```python
from build123d import *

# Parameters (mm, degrees)
SKETCH1_W              = 200
SKETCH1_H              = 50
BOSS_EXTRUDE1_DEPTH    = 7.5
CUT_EXTRUDE1_DEPTH     = 105.16333328
SHELL2_T               = -2
F_20_0MM_DOWEL_HOLE1_D = 2.9


with BuildPart() as part:
    # Sketch1 → Boss-Extrude1 (new, symmetric)
    with BuildSketch(Plane.XY):
        Rectangle(SKETCH1_W, SKETCH1_H)
    extrude(amount=BOSS_EXTRUDE1_DEPTH, both=True)

    # Sketch15 → Cut-Extrude1 (cut, through all)
    with BuildSketch(Plane(origin=(0, 0, -7.5), x_dir=(-1, 0, 0), z_dir=(0, 0, -1))):
        Polygon((-100.000000026, 0.510192391), (-100, 25), (100, 25), (100.000000026, 0.510192391), (0, 20.08555215), align=None)
        Polygon((-100.000000029, -0.965448702), (-100, -25), (100, -25), (100, -0.965448702), (0, -20.08535521), align=None)
    extrude(amount=-CUT_EXTRUDE1_DEPTH, mode=Mode.SUBTRACT)

    # Shell2
    shell2_openings = [part.faces().sort_by_distance(p)[0] for p in [
        (4e-09, -0.078500046, -7.5),
    ]]
    offset(amount=SHELL2_T, openings=shell2_openings)

    # Ø20.0mm Dowel Hole1 (through all)
    with Locations(Plane.XY.offset(7.5)):
        with Locations((-11.490485194, 11.490485194), (11.490485194, -11.490485194), (11.490485194, 11.490485194), (-11.490485194, -11.490485194)):
            Hole(F_20_0MM_DOWEL_HOLE1_D / 2)


solid = part.part
```
Model file for the job. Use its own axes, mm. A direction names the side the tool comes from. Give positions to 0.01 mm unless a question says otherwise; leave off trailing zeros. Write each loop counter-clockwise with the first axis right and the second up, starting at its lowest first coordinate (ties: lowest second). Pieces come first, ordered by that corner, then holes. Notation, with made-up numbers: M 22.5,84.5 L 47.5,84.5 A20 cw 47.5,91.5 Z; hole C 8,36 d11. An arc over 180 degrees is marked long. Use a Markdown table: item, result.
1) Tool access for faces 4 (the flat face through (-1, 0, 7.5)), 5 (the flat face through (-47.295, -9.006, -1.091)): list every direction of +Z, -Z, +X, -X, +Y, -Y with a clear straight run to the whole face (end or side of a thin tool).
Responses:
| item | result |
|---|---|
| face 4 | +Z, +X, -X, +Y, -Y |
| face 5 | -Z |
2) Cut at B-B (y = 2.5). List the corners of the cut face in (x, z).
Responses:
| item | result |
|---|---|
| outline | M -89.84,-7.5 L -79.42,-7.5 L -79.42,5.5 L 79.42,5.5 L 79.42,-7.5 L 89.84,-7.5 L 89.84,7.5 L -89.84,7.5 Z |
3) Pin check, flat tips, straight feed: pin 1 (2 mm diameter, centred on x = 39.5, z = 0, fed in from +Y); pin 2 (1.7 mm diameter, centred on x = 11.49, y = 11.49, fed in from +Z); pin 3 (4.5 mm diameter, centred on x = -11.49, y = -11.49, fed in from -Z); pin 4 (3 mm diameter, centred on x = -10.5, z = 3.5, fed in from +Y). Stop position of each tip, or through.
Responses:
| item | result |
|---|---|
| pin 1 | stops at y = 12.55 |
| pin 2 | passes through |
| pin 3 | stops at z = 5.5 |
| pin 4 | stops at y = 18.32 |
4) Pull direction X, two halves, no side cores. Call faces 1 (the flat face through (-50.7, 10.16, -0.11)), 2 (the flat face through (-1, 0, 5.5)), 3 (the flat face through (7, -18, -7.5)): +X half, -X half, draft (parallel to the pull), parting line (faces both ways), or undercut.
Responses:
| item | result |
|---|---|
| face 1 | -X half |
| face 2 | undercut |
| face 3 | draft |
5) Cut at C-C (x = 29). List the corners of the cut face in (y, z).
Responses:
| item | result |
|---|---|
| outline | M -14.54,-7.5 L -12.5,-7.5 L -12.5,5.5 L 12.37,5.5 L 12.37,-7.5 L 14.41,-7.5 L 14.41,7.5 L -14.54,7.5 Z |
6) Cut at A-A (z = -0.5). List the corners of the cut face in (x, y).
Responses:
| item | result |
|---|---|
| outline | M -100,-0.97 L 0,-20.09 L 100,-0.97 L 100,0.51 L 0,20.09 L -100,0.51 Z; hole M -93.28,-0.21 L 0,-18.05 L 93.28,-0.21 L 0,18.05 Z |
7) Drill centre lines: line 1 (Z direction, x = 20, y = -6.5); line 2 (Y direction, x = 84, z = -4); line 3 (Y direction, x = -60, z = -6). Where is each one in solid material? Low to high. Write a range as from..to.
Responses:
| item | result |
|---|---|
| line 1 | z = 5.5..7.5 |
| line 2 | y = -4.02..-1.99, 1.6..3.64 |
| line 3 | y = -8.61..-6.58, 6.3..8.34 |
